Check sheet for the modelled part. Datum: model origin and axes. Units: mm. A direction names the side the tool comes from. Give positions to 0.01 mm unless a question says otherwise; leave off trailing zeros. Order: outer loops, then holes, each group sorted by start corner. A loop starts at its lowest first (then second) coordinate and runs counter-clockwise, first axis right, second up. Notation, with made-up numbers: (47.5, -15.75) -> (105.5, -15.75) arc R3 ccw to (105.5, -10.75) -> close; hole circle Ø5 at (-30, 89.5). An arc over 180 degrees is marked (long way). One line per question, with ' | ' between items.
```python
from build123d import *

# Parameters (mm, degrees)
ESBO_O1_W                              = 126.1
ESBO_O1_H                              = 10
RESSALTO_EXTRUS_O1_DEPTH               = 10
CORTE_EXTRUS_O1_DEPTH                  = 65.033604459
CORTE_EXTRUS_O3_DEPTH                  = 3
ESBO_O4_R                              = 3
CORTE_EXTRUS_O4_DEPTH                  = 4
ESBO_O5_R                              = 1.25
CORTE_EXTRUS_O5_DEPTH                  = 65.11943933
CORTE_EXTRUS_O9_REACH                  = 66.034
CORTE_EXTRUS_O9_END_RADIUS             = 3
ESBO_O6_R                              = 1.5
CORTE_EXTRUS_O9_DIRECTION_2_REACH      = 66.034
CORTE_EXTRUS_O9_DIRECTION_2_END_RADIUS = 3
FILETE1_R                              = 3
FILETE2_R                              = 3


with BuildPart() as part:
    # Esboço1 → Ressalto-extrusão1 (new body)
    with BuildSketch(Plane.XY):
        Rectangle(ESBO_O1_W, ESBO_O1_H)
    extrude(amount=RESSALTO_EXTRUS_O1_DEPTH)

    # Esboço2 → Corte-extrusão1 (cut, through all)
    with BuildSketch(Plane.XY.offset(10)):
        with BuildLine():
            Line((-291.82946292, -50.413684991), (-53.05, -5))
            ThreePointArc((-53.05, -5), (0, 0), (53.05, -5))
            Line((53.05, -5), (291.82946292, -50.413684991))
            Line((291.82946292, -50.413684991), (291.82946292, -536.533154655))
            Line((291.82946292, -536.533154655), (-291.82946292, -536.533154655))
            Line((-291.82946292, -536.533154655), (-291.82946292, -50.413684991))
        make_face()
    extrude(amount=-CORTE_EXTRUS_O1_DEPTH, mode=Mode.SUBTRACT)

    # Esboço3 → Corte-extrusão3 (cut)
    with BuildSketch(Plane(origin=(0, -5, 0), x_dir=(1, 0, 0), z_dir=(0, 1, 0))):
        Polygon((-56.354018507, -7.946802806), (-54.650003164, -5.004638346), (-56.345984657, -2.05783554), (-59.745981493, -2.053197194), (-61.449996836, -4.995361654), (-59.754015343, -7.94216446), align=None)
    corte_extrus_o3 = extrude(amount=CORTE_EXTRUS_O3_DEPTH, mode=Mode.SUBTRACT)

    # Esboço4 → Corte-extrusão4 (cut)
    with BuildSketch(Plane(origin=(0, 5, 0), x_dir=(1, 0, 0), z_dir=(0, 1, 0))):
        with Locations(Location((-58.05, -5, 0), (0, 0, 270))):
            Circle(ESBO_O4_R)
    corte_extrus_o4 = extrude(amount=-CORTE_EXTRUS_O4_DEPTH, mode=Mode.SUBTRACT)

    # Esboço5 → Corte-extrusão5 (cut, through all)
    with BuildSketch(Plane(origin=(0, 1, 0), x_dir=(1, 0, 0), z_dir=(0, 1, 0))):
        with Locations(Location((-58.05, -5, 0), (0, 0, 270))):
            Circle(ESBO_O5_R)
    corte_extrus_o5 = extrude(amount=-CORTE_EXTRUS_O5_DEPTH, mode=Mode.SUBTRACT)

    # Espelhar2: Corte-extrusão3, Corte-extrusão4, Corte-extrusão5 across plane
    add(corte_extrus_o3.mirror(Plane(origin=(0, 0, 0), x_dir=(0, 0, 1), z_dir=(1, 0, 0))), mode=Mode.SUBTRACT)
    add(corte_extrus_o4.mirror(Plane(origin=(0, 0, 0), x_dir=(0, 0, 1), z_dir=(1, 0, 0))), mode=Mode.SUBTRACT)
    add(corte_extrus_o5.mirror(Plane(origin=(0, 0, 0), x_dir=(0, 0, 1), z_dir=(1, 0, 0))), mode=Mode.SUBTRACT)

    # Corte-extrusão9: up to this cylinder (the profile starts outside it)
    corte_extrus_o9_end = Plane(origin=(58.05, 3, 5), z_dir=(0, 1, 0)) * Cylinder(CORTE_EXTRUS_O9_END_RADIUS, 139.068, mode=Mode.PRIVATE)
    # Esboço6 → Corte-extrusão9 (cut, up to the surface)
    with BuildSketch(Plane.ZY, mode=Mode.PRIVATE) as corte_extrus_o9_sk1:
        with Locations(Location((5, 3, 0), (0, 0, 180))):
            Circle(ESBO_O6_R)
    corte_extrus_o9_tool1 = extrude(corte_extrus_o9_sk1.sketch, amount=-CORTE_EXTRUS_O9_REACH, mode=Mode.PRIVATE) - corte_extrus_o9_end
    add(corte_extrus_o9_tool1.solids().sort_by_distance((0, 3, 5))[0], mode=Mode.SUBTRACT)

    # Corte-extrusão9 direction 2: up to this cylinder (the profile starts outside it)
    corte_extrus_o9_direction_2_end = Plane(origin=(-58.05, 3, 5), z_dir=(0, 1, 0)) * Cylinder(CORTE_EXTRUS_O9_DIRECTION_2_END_RADIUS, 139.068, mode=Mode.PRIVATE)
    # Esboço6 → Corte-extrusão9 direction 2 (cut, up to the surface)
    with BuildSketch(Plane.ZY, mode=Mode.PRIVATE) as corte_extrus_o9_direction_2_sk1:
        with Locations(Location((5, 3, 0), (0, 0, 180))):
            Circle(ESBO_O6_R)
    corte_extrus_o9_direction_2_tool1 = extrude(corte_extrus_o9_direction_2_sk1.sketch, amount=CORTE_EXTRUS_O9_DIRECTION_2_REACH, mode=Mode.PRIVATE) - corte_extrus_o9_direction_2_end
    add(corte_extrus_o9_direction_2_tool1.solids().sort_by_distance((0, 3, 5))[0], mode=Mode.SUBTRACT)

    # Filete1
    # the kernel refuses this fillet: 3 mm, written as the material it takes off along each edge
    with BuildSketch(Plane(origin=(-63.05, 12.5, 10), x_dir=(1, 0, 0), z_dir=(0, -1, 0)), Plane(origin=(-63.05, 12.5, 0), x_dir=(0, 0, 1), z_dir=(0, -1, 0)), Plane(origin=(63.05, -12.5, 0), x_dir=(0, 0, 1), z_dir=(0, 1, 0)), Plane(origin=(-63.05, 5, -7.5), x_dir=(1, 0, 0), z_dir=(0, 0, 1)), Plane(origin=(63.05, 5, -7.5), x_dir=(0, -1, 0), z_dir=(0, 0, 1))) as filete1_piece_1:
        with BuildLine():
            CenterArc((FILETE1_R, -FILETE1_R), FILETE1_R, 90, 90)
            Line((0, -FILETE1_R), (0, 0))
            Line((0, 0), (FILETE1_R, 0))
        make_face()
    extrude(amount=25, mode=Mode.SUBTRACT)
    with BuildSketch(Plane(origin=(63.05, -12.5, 10), x_dir=(0, 0, -1), z_dir=(0, 1, 0))) as filete1_piece_2:
        with BuildLine():
            CenterArc((FILETE1_R, FILETE1_R), FILETE1_R, 180, 90)
            Line((0, FILETE1_R), (0, 0))
            Line((0, 0), (FILETE1_R, 0))
        make_face()
    extrude(amount=25, mode=Mode.SUBTRACT)

    # Filete2
    # the kernel refuses this fillet: 3 mm, written as the material it takes off along each edge
    with BuildSketch(Plane(origin=(45.55, -5, 0), x_dir=(0, 1, 0), z_dir=(1, 0, 0)), Plane(origin=(-60.05, -5, 10), x_dir=(0, 0, -1), z_dir=(1, 0, 0))) as filete2_piece_1:
        with BuildLine():
            CenterArc((FILETE2_R, FILETE2_R), FILETE2_R, 180, 90)
            Line((0, FILETE2_R), (0, 0))
            Line((0, 0), (FILETE2_R, 0))
        make_face()
    extrude(amount=14.5, mode=Mode.SUBTRACT)
    with BuildSketch(Plane(origin=(45.55, -5, 10), x_dir=(0, 1, 0), z_dir=(1, 0, 0)), Plane(origin=(-60.05, -5, 0), x_dir=(0, 0, 1), z_dir=(1, 0, 0))) as filete2_piece_2:
        with BuildLine():
            CenterArc((FILETE2_R, -FILETE2_R), FILETE2_R, 90, 90)
            Line((0, -FILETE2_R), (0, 0))
            Line((0, 0), (FILETE2_R, 0))
        make_face()
    extrude(amount=14.5, mode=Mode.SUBTRACT)
    with BuildSketch(Plane(origin=(0, -283.93025, 0), x_dir=(0.21272383034714434, 0.9771123640617998, 0), z_dir=(0.9771123640617998, -0.21272383034714434, 0))) as filete2_piece_3:
        with BuildLine():
            CenterArc((283.93025 + FILETE2_R, FILETE2_R), FILETE2_R, 180, 90)
            Line((283.93025, FILETE2_R), (283.93025, 0))
            Line((283.93025, 0), (283.93025 + FILETE2_R, 0))
        make_face()
    revolve(axis=Axis((0, -283.93025, 0), (0, 0, 1)), revolution_arc=24.564047203, mode=Mode.SUBTRACT)
    with BuildSketch(Plane(origin=(0, -283.93025, 10), x_dir=(-0.21272383034714376, 0.9771123640618, 0), z_dir=(-0.9771123640618, -0.21272383034714376, 0))) as filete2_piece_4:
        with BuildLine():
            CenterArc((283.93025 + FILETE2_R, FILETE2_R), FILETE2_R, 180, 90)
            Line((283.93025 + FILETE2_R, 0), (283.93025, 0))
            Line((283.93025, 0), (283.93025, FILETE2_R))
        make_face()
    revolve(axis=Axis((0, -283.93025, 10), (0, 0, -1)), revolution_arc=24.564047203, mode=Mode.SUBTRACT)
    with BuildSketch(Plane(origin=(-60.05, -5, 3), x_dir=(0, 0, -1), z_dir=(1, 0, 0))) as filete2_piece_5:
        with BuildLine():
            CenterArc((3 - FILETE2_R, FILETE2_R), FILETE2_R, 270, 90)
            Line((3, FILETE2_R), (3, 0))
            Line((3, 0), (3 - FILETE2_R, 0))
        make_face()
    revolve(axis=Axis((-60.05, -5, 3), (0, 1, 0)), revolution_arc=90, mode=Mode.SUBTRACT)
    with BuildSketch(Plane(origin=(-63.05, -5, 3), x_dir=(1, 0, 0), z_dir=(0, 0, 1))) as filete2_piece_6:
        with BuildLine():
            CenterArc((FILETE2_R, FILETE2_R), FILETE2_R, 180, 90)
            Line((0, FILETE2_R), (0, 0))
            Line((0, 0), (FILETE2_R, 0))
        make_face()
    extrude(amount=4, mode=Mode.SUBTRACT)
    with BuildSketch(Plane(origin=(-60.05, -5, 7), x_dir=(-1, 0, 0), z_dir=(0, 0, -1))) as filete2_piece_7:
        with BuildLine():
            CenterArc((3 - FILETE2_R, FILETE2_R), FILETE2_R, 270, 90)
            Line((3, FILETE2_R), (3, 0))
            Line((3, 0), (3 - FILETE2_R, 0))
        make_face()
    revolve(axis=Axis((-60.05, -5, 7), (0, 1, 0)), revolution_arc=90, mode=Mode.SUBTRACT)
    with BuildSketch(Plane(origin=(60.05, -5, 7), x_dir=(1, 0, 0), z_dir=(0, 0, -1))) as filete2_piece_8:
        with BuildLine():
            CenterArc((3 - FILETE2_R, -FILETE2_R), FILETE2_R, 0, 90)
            Line((3, -FILETE2_R), (3, 0))
            Line((3, 0), (3 - FILETE2_R, 0))
        make_face()
    revolve(axis=Axis((60.05, -5, 7), (0, -1, 0)), revolution_arc=90, mode=Mode.SUBTRACT)
    with BuildSketch(Plane(origin=(63.05, -5, 3), x_dir=(-1, 0, 0), z_dir=(0, 0, 1))) as filete2_piece_9:
        with BuildLine():
            CenterArc((FILETE2_R, -FILETE2_R), FILETE2_R, 90, 90)
            Line((0, -FILETE2_R), (0, 0))
            Line((0, 0), (FILETE2_R, 0))
        make_face()
    extrude(amount=4, mode=Mode.SUBTRACT)
    with BuildSketch(Plane(origin=(60.05, -5, 3), x_dir=(0, 0, -1), z_dir=(-1, 0, 0))) as filete2_piece_10:
        with BuildLine():
            CenterArc((3 - FILETE2_R, -FILETE2_R), FILETE2_R, 0, 90)
            Line((3 - FILETE2_R, 0), (3, 0))
            Line((3, 0), (3, -FILETE2_R))
        make_face()
    revolve(axis=Axis((60.05, -5, 3), (0, -1, 0)), revolution_arc=90, mode=Mode.SUBTRACT)


solid = part.part
```
Q1. Depth check by flat-ended pin: pin 1 Ø2 at (x, y) = (26, -1) entering from -Z; pin 2 Ø1.8 at (x, z) = (-57, 5) entering from +Y; pin 3 Ø1.5 at (y, z) = (3, 8.5) entering from +X; pin 4 Ø1.5 at (x, z) = (58.05, 5) entering from -Y. Enter the tip coordinate at first touch or a pass-through.
Result sheet:
pin 1: stops at z = 0.61 | pin 2: stops at y = 1 | pin 3: stops at x = 62.95 | pin 4: passes through
Q2. Section check A-A (x = 58.05). Enter the section's corners in (y, z).
Result sheet:
outline: (-4.85, 2.06) arc R3 ccw to (-2, 0) -> (5, 0) -> (5, 2) -> (1, 2) -> (1, 3.75) -> (-2, 3.75) -> (-2, 2.06) -> close; (-4.85, 7.94) -> (-2, 7.94) -> (-2, 6.25) -> (1, 6.25) -> (1, 8) -> (5, 8) -> (5, 10) -> (-2, 10) arc R3 ccw to start
Q3. Mould release check, pull along X, two halves, no side actions. Record for faces 3 (the face through (-1, 5, 5)), 4 (the face through (-56.6, -2, 5)), 5 (the face through (-63.05, 0, 5)), 6 (the face through (56.6, -2, 5)): pulls with the +X half, pulls with the -X half, needs draft (parallel to the pull), parting line crosses it, or undercut.
Result sheet:
face 3: needs draft | face 4: undercut | face 5: pulls with the -X half | face 6: undercut
Q4. Thickness scan on line 1 (Z direction, x = 58.05, y = 2.6); line 2 (X direction, y = 2.5, z = 7.25); line 3 (Z direction, x = 58.05, y = -0.45). Record the ranges inside material, lowest first.
Result sheet:
line 1: z = 0 to 2, 8 to 10 | line 2: x = -63.01 to -60.03, -56.07 to 56.07, 60.03 to 63.01 | line 3: z = 0 to 3.75, 6.25 to 10
Q5. Access from +Z, -Z, +X, -X, +Y, -Y to the whole of each face (thin tool, end or side, straight path). Record for faces 1 (the face through (55.486, -3.521, 3.552)), 2 (the face through (59.27, -0.48, 4.73)).
Result sheet:
face 1: -Y | face 2: +Y, -Y
